Check sheet for the drawn part. Datum: minimum x, y, z corner. Units: mm. A direction names the side the tool comes from. Coordinates: 2 decimals unless noted, no trailing zeros. Write each loop counter-clockwise with the first axis right and the second up, starting at its lowest first coordinate (ties: lowest second). Pieces come first, ordered by that corner, then holes. Notation, with made-up numbers: (-9, 9.5) -> (44, 9.5) arc R17 cw to (44, 40.5) -> close; hole circle Ø7 at (31.25, 18). An arc over 180 degrees is marked (long way). One line per question, with ' | ' between items.
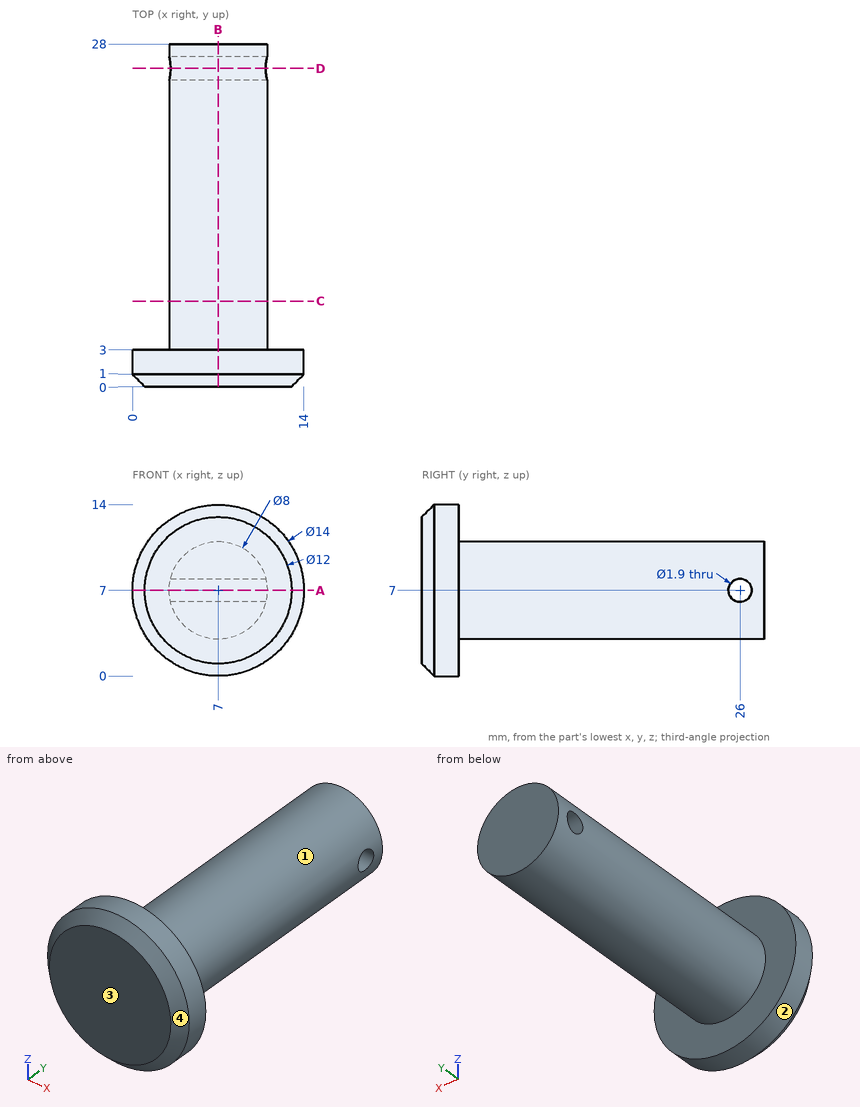
1. Cross-section at A-A on z = 7. Record the boundary of the cut face in (x, y).
Worked answers:
outline: (0, 1) -> (1, 0) -> (13, 0) -> (14, 1) -> (14, 3) -> (11, 3) -> (11, 25.05) -> (3, 25.05) -> (3, 3) -> (0, 3) -> close; (3, 26.95) -> (11, 26.95) -> (11, 28) -> (3, 28) -> close
2. Cross-section at C-C on y = 7. Record the boundary of the cut face in (x, z), and give its area (3 significant figures).
Worked answers:
outline: circle Ø8 at (7, 7) | area: 50.3 mm²
3. Material ranges on line 1 (Y direction, x = 8, z = 7); line 2 (Y direction, x = 3.25, z = 5.25); line 3 (Z direction, x = 5.75, y = 26), recorded low to high. Write a range as from..to.
Worked answers:
line 1: 0..25.05, 26.95..28 | line 2: 0..3 | line 3: 3.2..6.05, 7.95..10.8
4. Cross-section at D-D on y = 26. Record the boundary of the cut face in (x, z), and give its area (3 significant figures).
Worked answers:
outline: (3.11, 6.05) arc R4 ccw to (10.89, 6.05) -> close; (3.11, 7.95) -> (10.89, 7.95) arc R4 ccw to start | area: 35.2 mm²
5. Mould release check, pull along Z, two halves, no side actions. Record for the marked faces 3 and 4: released by +Z, released by -Z, zero draft, split by the parting line, or undercut.
Worked answers:
face 3: zero draft | face 4: split by the parting line
6. Tool access check on the marked faces 1 and 2. Record the directions out of +Z, -Z, +X, -X, +Y, -Y that give a thin tool (end or side, any length) a straight path to the whole face; none if there is none.
Worked answers:
face 1: +Y | face 2: +Y, -Y
7. Go/stop test with flat-tipped pins: P1, Ø5, axis at x = 1.5, y = 17, coming from the +Z side; P2, Ø2, axis at x = 7.5, z = 2.5, coming from the +Y side; P3, Ø3, axis at y = 26, z = 7, coming from the -X side; P4, Ø8, axis at y = 13.5, z = 2, coming from the +X side. Record where each tip stops, or that it passes through.
Worked answers:
P1: z = 9.65 | P2: y = 28 | P3: x = 3 | P4: x = 10.87
8. Cross-section at B-B on x = 7. Record the boundary of the cut face in (y, z).
Worked answers:
outline: (0, 1) -> (1, 0) -> (3, 0) -> (3, 3) -> (28, 3) -> (28, 11) -> (3, 11) -> (3, 14) -> (1, 14) -> (0, 13) -> close; hole circle Ø1.9 at (26, 7)
